Can you work these out from the model? Positions are in its coordinate system, mm. A direction names the side the tool comes from. Round coordinates to 2 decimals unless told otherwise and drop trailing zeros. Write each loop counter-clockwise with the first axis right and the second up, starting at its lowest first coordinate (ties: lowest second). Pieces come first, ordered by that corner, then holes. Notation, with made-up numbers: (18, -38) -> (28, -38) arc R30 ccw to (28, -3) -> close; hole circle Ø4 at (-30.5, -14). An arc over 180 degrees is marked (long way). Write item = value, one per line. Start each with the question number.
1) Imagine slicing it at C-C, the plane z = 4.75. Please give me the cut outline in (x, y), then the cut area to 3 significant figures.
2) Imagine slicing it at B-B, the plane x = 0. Please give me the cut outline in (y, z), then the cut area to 3 significant figures.
3) Imagine slicing it at A-A, the plane y = 0. Please give me the cut outline in (x, z), then the cut area to 3 significant figures.
4) If I drill on line 1 (Y direction, x = 0, z = -11); line 2 (Y direction, x = 0, z = -1.3); line 3 (Y direction, x = 2.75, z = -0.75), over which ranges is the centre line in solid material (lowest first)?
5) Thinking about a two-plate mould opening in Y: for faces 1 (the face through (-1.73, -7.81, -8.57)), 2 (the face through (-2.17, -9.76, 0.18)), which applies, +Y half, -Y half, draft (parallel to the pull), parting line (faces both ways), or undercut?
6) For faces 3 (the face through (-1.73, -7.81, 6.91)), 4 (the face through (-4.57, 7.167, -1.528)), which set-ups out of +Z, -Z, +X, -X, +Y, -Y let a thin tool reach every point of the face, with its end or its side?
7) I'm going to push flat-ended pins straight in: pin 1 (3 mm diameter, centred on x = -2.5, z = -1, fed in from -Y); pin 2 (6 mm diameter, centred on x = 8, z = -2, fed in from -Y). Where does each tip first touch, or does it pass through?
from build123d import *

# Parameters (mm, degrees)
SKETCH_1_R          = 10
SKETCH_1_R_2        = 8
EXTRUDE_1_DEPTH     = 13.5
CHAMFER_1_SIZE      = 1
CUT_EXTRUDE_START   = -10
SKETCH_2_R          = 8.5
CUT_EXTRUDE_1_DEPTH = 4
SWEEP_1_PROFILE_R   = 1


with BuildPart() as part:
    # 草图1 → 凸台-拉伸1 (new, symmetric)
    with BuildSketch(Plane.XY):
        Circle(SKETCH_1_R)
        Circle(SKETCH_1_R_2, mode=Mode.SUBTRACT)
    extrude(amount=EXTRUDE_1_DEPTH, both=True)

    # 倒角1
    chamfer_1_edges = [part.edges().sort_by_distance(p)[0] for p in [
        (-10, 0, -13.5),
        (-10, 0, 13.5),
    ]]
    chamfer(chamfer_1_edges, length=CHAMFER_1_SIZE)

    # 草图2 → 切除-拉伸1 (cut)
    with BuildSketch(Plane(origin=(0, 0, -13.5), x_dir=(-1, 0, 0), z_dir=(0, 0, -1)).offset(CUT_EXTRUDE_START)):
        Circle(SKETCH_2_R)
    extrude(amount=-CUT_EXTRUDE_1_DEPTH, mode=Mode.SUBTRACT)

    # 切除-扫描1: sweep along a path in 草图3
    with BuildLine(Plane(origin=(0, 0, 0), x_dir=(0, 0, -1), z_dir=(1, 0, 0))) as sweep_1_path:
        Line((5.960249648, 12.918859865), (1.5, 8.458610217))
        Line((1.5, 8.458610217), (-2.960249648, 12.918859865))
    # 切除-扫描1 profile (on start of the path) → 切除-扫描1 (sweep, cut)
    with BuildSketch(Plane(origin=(0, 12.918859865, -5.960249648), x_dir=(0, 0.7071067811865478, 0.7071067811865472), z_dir=(0, -0.7071067811865472, 0.7071067811865478))):
        Circle(SWEEP_1_PROFILE_R)
    sweep(path=sweep_1_path.line, transition=Transition.RIGHT, mode=Mode.SUBTRACT)


solid = part.part
Reported:
q1.outline = circle Ø20 at (0, 0); hole circle Ø16 at (0, 0)
q1.area = 113 mm²
q2.outline = (-10, -12.5) -> (-9, -13.5) -> (-8, -13.5) -> (-8, -3.5) -> (-8.5, -3.5) -> (-8.5, 0.5) -> (-8, 0.5) -> (-8, 13.5) -> (-9, 13.5) -> (-10, 12.5) -> close; (8, -13.5) -> (9, -13.5) -> (10, -12.5) -> (10, -4.46) -> (8.5, -2.96) -> (8.5, -3.5) -> (8, -3.5) -> close; (8, 0.5) -> (8.5, 0.5) -> (8.5, -0.04) -> (10, 1.46) -> (10, 12.5) -> (9, 13.5) -> (8, 13.5) -> close; (9.87, -1.5) -> (10, -1.63) -> (10, -1.37) -> close
q2.area = 95.4 mm²
q3.outline = (-10, -12.5) -> (-9, -13.5) -> (-8, -13.5) -> (-8, -3.5) -> (-8.5, -3.5) -> (-8.5, 0.5) -> (-8, 0.5) -> (-8, 13.5) -> (-9, 13.5) -> (-10, 12.5) -> close; (8, -13.5) -> (9, -13.5) -> (10, -12.5) -> (10, 12.5) -> (9, 13.5) -> (8, 13.5) -> (8, 0.5) -> (8.5, 0.5) -> (8.5, -3.5) -> (8, -3.5) -> close
q3.area = 102 mm²
q4.line_1 = -10 to -8, 8 to 10
q4.line_2 = -10 to -8.5
q4.line_3 = -9.61 to -8.04, 8.04 to 9.61
q5.face_1 = undercut
q5.face_2 = parting line
q6.face_3 = +Z, -Z
q6.face_4 = none
q7.pin_1 = -9.95
q7.pin_2 = -8.66
